Check sheet for the modelled part. Datum: model origin and axes. Units: mm. A direction names the side the tool comes from. Give positions to 0.01 mm unless a question says otherwise; leave off trailing zeros. Write each loop counter-clockwise with the first axis right and the second up, starting at its lowest first coordinate (ties: lowest second). Pieces come first, ordered by that corner, then holes. Notation, with made-up numbers: (29, 4) -> (63, 4) arc R25 ccw to (63, 19) -> close; hole circle Ø3 at (-36.5, 69.25). An arc over 180 degrees is marked (long way). Return JSON: item names as keys, results as strings.
Autodesk Inventor part; units mm, degrees
ref_plane "YZ Plane" through (0, 0, 0) normal (1, 0, 0) x (0, 1, 0)
ref_plane "XZ Plane" through (0, 0, 0) normal (0, 1, 0) x (-1, 0, 0)
ref_plane "XY Plane" through (0, 0, 0) normal (0, 0, 1) x (1, 0, 0)
sketch "Sketch2" plane through (0, 0, 0) normal (0, 1, 0) x (-1, 0, 0)
  line L0 (0, 0) -> (5.5, 0)
  line L1 (5.5, 0) -> (5.5, 3)
  line L2 (5.5, 3) -> (0, 3)
  line L3 (0, 3) -> (0, 0)
  line L4 (5.5, 3) -> (-6.7, 3)
  line L5 (-6.7, 3) -> (-6.7, -3.1)
  line L6 (-6.7, -3.1) -> (5.5, -3.1)
  line L7 (5.5, -3.1) -> (5.5, 3)
  dimension "d0" = 5.5
  dimension "d1" = 3
  dimension "d2" = 12.2
  dimension "d3" = 6.1
extrude "Extrusion1" add sketch "Sketch2" along normal blind 7.5
sketch "Sketch3" plane through (0, 7.5, 0) normal (0, 1, 0) x (1, 0, 0)
  line L0 (6.2, 2.1) -> (-5, 2.1)
  line L1 (-5, 2.1) -> (-5, -3.6)
  line L2 (-5, -3.6) -> (6.2, -3.6)
  line L3 (6.2, -3.6) -> (6.2, 2.1)
  line L4 (6.7, 3.1) -> (-5.5, 3.1)
  line L5 (6.7, -3) -> (6.7, 3.1)
  point P0 (0, 0)
  dimension "d6" = 6.7
  dimension "d7" = 5.7
  dimension "d8" = 11.2
  dimension "d9" = 0.5
extrude "Extrusion2" add sketch "Sketch3" along normal blind 43.5
sketch "Sketch4" plane through (0, 0, 0) normal (0, -1, 0) x (1, 0, 0)
  line L0 (-1.45, -1.9) -> (2.65, -1.9)
  line L1 (2.65, -1.9) -> (2.65, 1.3)
  line L2 (2.65, 1.3) -> (-1.45, 1.3)
  line L3 (-1.45, 1.3) -> (-1.45, -1.9)
  line L4 (-5.5, 3) -> (6.7, 3)
  line L5 (-5.5, -3.1) -> (-5.5, 3)
  point P0 (0, 0)
  dimension "d12" = 3.2
  dimension "d13" = 4.1
  dimension "d14" = 1.7
  dimension "d15" = 4.05
extrude "Extrusion3" add sketch "Sketch4" along normal blind 9.5
properties part number "Battery_small"
(1) Depth check by flat-ended pin: pin 1 Ø3 at (y, z) = (25.5, 0.5) entering from -X; pin 2 Ø2 at (x, y) = (0, 2.5) entering from +Z; pin 3 Ø3 at (y, z) = (36.5, 1.5) entering from +X. Enter the tip coordinate at first touch or a pass-through.
Reply:
{"pin 1": "x = -5", "pin 2": "z = 3", "pin 3": "x = 6.2"}
(2) Cross-section at A-A on z = -0.25. Enter the section's corners in (x, y), then the cut area to 3 significant figures.
Reply:
{"outline": "(-5.5, 0) -> (-1.45, 0) -> (-1.45, -9.5) -> (2.65, -9.5) -> (2.65, 0) -> (6.7, 0) -> (6.7, 7.5) -> (6.2, 7.5) -> (6.2, 51) -> (-5, 51) -> (-5, 7.5) -> (-5.5, 7.5) -> close", "area": "618 mm^2"}
(3) Set-up check for faces 1 (the flat face through (6.2, 29, 1)), 2 (the flat face through (1, 29, -2.1)), 3 (the flat face through (-5, 29, 1)), 4 (the flat face through (1, -5, 1.3)), 5 (the flat face through (1, -5, -1.9)): record each of +Z, -Z, +X, -X, +Y, -Y from which the full face is reachable in a straight line by a thin tool's end or side.
Reply:
{"face 1": "+Z, -Z, +X, +Y", "face 2": "-Z, +X, -X, +Y", "face 3": "+Z, -Z, -X, +Y", "face 4": "+Z, +X, -X, -Y", "face 5": "-Z, +X, -X, -Y"}
(4) Cross-section at D-D on x = 4.25. Enter the section's corners in (y, z).
Reply:
{"outline": "(0, -3.1) -> (7.5, -3.1) -> (7.5, -2.1) -> (51, -2.1) -> (51, 3.6) -> (7.5, 3.6) -> (7.5, 3) -> (0, 3) -> close"}
(5) Cross-section at B-B on x = 1.5. Enter the section's corners in (y, z).
Reply:
{"outline": "(-9.5, -1.9) -> (0, -1.9) -> (0, -3.1) -> (7.5, -3.1) -> (7.5, -2.1) -> (51, -2.1) -> (51, 3.6) -> (7.5, 3.6) -> (7.5, 3) -> (0, 3) -> (0, 1.3) -> (-9.5, 1.3) -> close"}
(6) Cross-section at C-C on y = 33. Enter the section's corners in (x, z).
Reply:
{"outline": "(-5, -2.1) -> (6.2, -2.1) -> (6.2, 3.6) -> (-5, 3.6) -> close"}
(7) Thickness scan on L1, parallel to Z at x = 3.5, y = 17.5; L2, parallel to Z at x = 0.75, y = 4; L3, parallel to X at y = 41.5, z = 3.25. Record the ranges inside material, lowest first.
Reply:
{"L1": "-2.1 to 3.6", "L2": "-3.1 to 3", "L3": "-5 to 6.2"}
